Here's how the part is built. I have some questions about the finished solid (model axes, mm). A direction names the side the tool comes from. Round coordinates to 2 decimals unless told otherwise and drop trailing zeros. Order: outer loops, then holes, each group sorted by start corner. A loop starts at its lowest first (then second) coordinate and runs counter-clockwise, first axis right, second up. Notation, with made-up numbers: (-12, -2.5) -> (10, -2.5) arc R19 cw to (10, 24.5) -> close; hole circle Ø6 at (72.5, 12.5). An arc over 180 degrees is marked (long way). One line per item, written item: value.
```python
from build123d import *

# Parameters (mm, degrees)
F1_DEPTH = 927.1
F3_DEPTH = 203.201


with BuildPart() as f1:
    # F0 (on Right) → F1 (new body, symmetric)
    with BuildSketch(Plane.YZ):
        with BuildLine():
            Line((64.1858, 101.6), (0, 101.6))
            Line((0, 101.6), (0, -101.6))
            Line((0, -101.6), (64.1858, -101.6))
            Line((64.1858, -101.6), (64.1858, -92.636418))
            ThreePointArc((64.1858, -92.636418), (63.339447, -90.478171), (61.251608, -89.470563))
            Line((61.251608, -89.470563), (23.161034, -86.573234))
            ThreePointArc((23.161034, -86.573234), (15.482479, -82.8675), (12.3698, -74.93))
            Line((12.3698, -74.93), (12.3698, 74.93))
            ThreePointArc((12.3698, 74.93), (15.482479, 82.8675), (23.161034, 86.573234))
            Line((23.161034, 86.573234), (61.251608, 89.470563))
            ThreePointArc((61.251608, 89.470563), (63.339447, 90.478171), (64.1858, 92.636418))
            Line((64.1858, 92.636418), (64.1858, 101.6))
        make_face()
    extrude(amount=F1_DEPTH, both=True)

    # F2 (on face) → F3 (cut, through all)
    with BuildSketch(Plane.XY.offset(101.6)):
        Polygon((-913.186131, 64.1858), (-927.1, 64.1858), (-927.1, 0), (-863.12883, 0), align=None)
        Polygon((927.1, 0), (927.1, 64.1858), (913.186131, 64.1858), (863.12883, 0), align=None)
    extrude(amount=-F3_DEPTH, mode=Mode.SUBTRACT)


solid = f1.part
```
Q1. If we mould it in two halves opening along Z, with no side actions, what happens to faces 3 (the face through (13, 33, 101.6)), 4 (the face through (12.8, 41.9, 88)), 5 (the face through (-871.121, 10.248, 1.422))? For each: pulls with the +Z half, pulls with the -Z half, needs draft (parallel to the pull), parting line crosses it, or undercut.
Answers:
face 3: pulls with the +Z half
face 4: undercut
face 5: needs draft
Q2. I need wall thicknesses on line 1 along Z through (x, y) = (674.5, 24); line 2 along Z through (x, y) = (836, 58.5); line 3 along Y through (x, z) = (690, -7.5). Which ranges of each line are inside material? Lowest first, please.
Answers:
line 1: -101.6 to -86.64, 86.64 to 101.6
line 2: -101.6 to -89.26, 89.26 to 101.6
line 3: 0 to 12.37
Q3. Which directions (+Z, -Z, +X, -X, +Y, -Y) give clear straight access to the entire face, cutting with the end or side of a thin tool? Please do faces 1 (the face through (12, 0, 1)), 2 (the face through (12, 12.37, -1)).
Answers:
face 1: +Z, -Z, +X, -X, -Y
face 2: +X, -X, +Y
Q4. I want a section at A-A on y = 41.5. Write out the boundary of the cut face in (x, z), then the cut area to 3 significant figures.
Answers:
outline: (-895.49, -101.6) -> (895.49, -101.6) -> (895.49, -87.97) -> (-895.49, -87.97) -> close; (-895.49, 87.97) -> (895.49, 87.97) -> (895.49, 101.6) -> (-895.49, 101.6) -> close
area: 48,800 mm2
Q5. I want a section at B-B on x = 417. Write out the boundary of the cut face in (y, z) (3 decimals).
Answers:
outline: (0, -101.6) -> (64.186, -101.6) -> (64.186, -92.636) arc R3.175 ccw to (61.252, -89.471) -> (23.161, -86.573) arc R11.677 cw to (12.37, -74.93) -> (12.37, 74.93) arc R11.677 cw to (23.161, 86.573) -> (61.252, 89.471) arc R3.175 ccw to (64.186, 92.636) -> (64.186, 101.6) -> (0, 101.6) -> close
Q6. I want a section at C-C on z = 31.5. Write out the boundary of the cut face in (x, y).
Answers:
outline: (-872.78, 12.37) -> (-863.13, 0) -> (863.13, 0) -> (872.78, 12.37) -> close
